from build123d import *

# Parameters (mm, degrees)
F0_R     = 6.35
F1_DEPTH = 12.7
F3_R     = 6.35
F4_DEPTH = 12.7


with BuildPart() as f1:
    # F0 (on Top) → F1 (new body)
    with BuildSketch(Plane.XY):
        with BuildLine():
            ThreePointArc((-163.4358839095, -121.5245512031), (-148.5569083937, -157.4455756873), (-112.6358839095, -172.3245512031))
            Line((-112.6358839095, -172.3245512031), (119.0192133605, -172.3245512031))
            ThreePointArc((119.0192133605, -172.3245512031), (154.9402378448, -157.4455756873), (169.8192133605, -121.5245512031))
            Line((169.8192133605, -121.5245512031), (169.8192133605, 115.6596517303))
            ThreePointArc((169.8192133605, 115.6596517303), (154.9402378448, 151.5806762145), (119.0192133605, 166.4596517303))
            Line((119.0192133605, 166.4596517303), (-112.6358839095, 166.4596517303))
            ThreePointArc((-112.6358839095, 166.4596517303), (-148.5569083937, 151.5806762145), (-163.4358839095, 115.6596517303))
            Line((-163.4358839095, 115.6596517303), (-163.4358839095, -121.5245512031))
        make_face()
        Polygon((-17.7260840714, -157.4455756873), (1.3239159286, -106.6455756873), (20.3739159286, -157.4455756873), align=None, mode=Mode.SUBTRACT)
        Polygon((-148.5569083937, -21.0277362994), (-148.5569083937, 17.0722637006), (-97.7569083937, 0.7111747481), align=None, mode=Mode.SUBTRACT)
        with Locations((1.3239159286, 0.7111747481)):
            Circle(F0_R, mode=Mode.SUBTRACT)
        Polygon((20.3739159286, 151.5806762145), (1.3239159286, 100.7806762145), (-17.7260840714, 151.5806762145), align=None, mode=Mode.SUBTRACT)
        Polygon((154.9402378448, -21.0277362994), (104.1402378448, 0.7111747481), (154.9402378448, 17.0722637006), align=None, mode=Mode.SUBTRACT)
    extrude(amount=F1_DEPTH)


with BuildPart() as f4:
    # F3 (on Top) → F4 (new body)
    with BuildSketch(Plane.XY):
        with BuildLine():
            ThreePointArc((-163.4358839095, -121.5245512031), (-148.5569083937, -157.4455756873), (-112.6358839095, -172.3245512031))
            Line((-112.6358839095, -172.3245512031), (119.0192133605, -172.3245512031))
            ThreePointArc((119.0192133605, -172.3245512031), (154.9402378448, -157.4455756873), (169.8192133605, -121.5245512031))
            Line((169.8192133605, -121.5245512031), (169.8192133605, 115.6596517303))
            ThreePointArc((169.8192133605, 115.6596517303), (154.9402378448, 151.5806762145), (119.0192133605, 166.4596517303))
            Line((119.0192133605, 166.4596517303), (-112.6358839095, 166.4596517303))
            ThreePointArc((-112.6358839095, 166.4596517303), (-148.5569083937, 151.5806762145), (-163.4358839095, 115.6596517303))
            Line((-163.4358839095, 115.6596517303), (-163.4358839095, -121.5245512031))
        make_face()
        with BuildLine():
            ThreePointArc((-68.5260840714, -21.0277362994), (-32.6050595871, -35.9067118152), (-17.7260840714, -71.8277362994))
            Line((-17.7260840714, -71.8277362994), (-17.7260840714, -106.6455756873))
            ThreePointArc((-17.7260840714, -106.6455756873), (-32.6050595871, -142.5666001716), (-68.5260840714, -157.4455756873))
            Line((-68.5260840714, -157.4455756873), (-97.7569083937, -157.4455756873))
            ThreePointArc((-97.7569083937, -157.4455756873), (-133.677932878, -142.5666001716), (-148.5569083937, -106.6455756873))
            Line((-148.5569083937, -106.6455756873), (-148.5569083937, -71.8277362994))
            ThreePointArc((-148.5569083937, -71.8277362994), (-133.677932878, -35.9067118152), (-97.7569083937, -21.0277362994))
            Line((-97.7569083937, -21.0277362994), (-68.5260840714, -21.0277362994))
        make_face(mode=Mode.SUBTRACT)
        Polygon((-17.7260840714, -157.4455756873), (1.3239159286, -106.6455756873), (20.3739159286, -157.4455756873), align=None, mode=Mode.SUBTRACT)
        with BuildLine():
            Line((71.1739159286, -21.0277362994), (104.1402378448, -21.0277362994))
            ThreePointArc((104.1402378448, -21.0277362994), (140.0612623291, -35.9067118152), (154.9402378448, -71.8277362994))
            Line((154.9402378448, -71.8277362994), (154.9402378448, -106.6455756873))
            ThreePointArc((154.9402378448, -106.6455756873), (140.0612623291, -142.5666001716), (104.1402378448, -157.4455756873))
            Line((104.1402378448, -157.4455756873), (71.1739159286, -157.4455756873))
            ThreePointArc((71.1739159286, -157.4455756873), (35.2528914443, -142.5666001716), (20.3739159286, -106.6455756873))
            Line((20.3739159286, -106.6455756873), (20.3739159286, -71.8277362994))
            ThreePointArc((20.3739159286, -71.8277362994), (35.2528914443, -35.9067118152), (71.1739159286, -21.0277362994))
        make_face(mode=Mode.SUBTRACT)
        Polygon((-148.5569083937, -21.0277362994), (-148.5569083937, 17.0722637006), (-97.7569083937, 0.7111747481), align=None, mode=Mode.SUBTRACT)
        with Locations((1.3239159286, 0.7111747481)):
            Circle(F3_R, mode=Mode.SUBTRACT)
        with BuildLine():
            ThreePointArc((-68.5260840714, 151.5806762145), (-32.6050595871, 136.7017006988), (-17.7260840714, 100.7806762145))
            Line((-17.7260840714, 100.7806762145), (-17.7260840714, 67.8722637006))
            ThreePointArc((-17.7260840714, 67.8722637006), (-32.6050595871, 31.9512392163), (-68.5260840714, 17.0722637006))
            Line((-68.5260840714, 17.0722637006), (-97.7569083937, 17.0722637006))
            ThreePointArc((-97.7569083937, 17.0722637006), (-133.677932878, 31.9512392163), (-148.5569083937, 67.8722637006))
            Line((-148.5569083937, 67.8722637006), (-148.5569083937, 100.7806762145))
            ThreePointArc((-148.5569083937, 100.7806762145), (-133.677932878, 136.7017006988), (-97.7569083937, 151.5806762145))
            Line((-97.7569083937, 151.5806762145), (-68.5260840714, 151.5806762145))
        make_face(mode=Mode.SUBTRACT)
        Polygon((20.3739159286, 151.5806762145), (1.3239159286, 100.7806762145), (-17.7260840714, 151.5806762145), align=None, mode=Mode.SUBTRACT)
        Polygon((154.9402378448, -21.0277362994), (104.1402378448, 0.7111747481), (154.9402378448, 17.0722637006), align=None, mode=Mode.SUBTRACT)
        with BuildLine():
            ThreePointArc((154.9402378448, 67.8722637006), (140.0612623291, 31.9512392163), (104.1402378448, 17.0722637006))
            Line((104.1402378448, 17.0722637006), (71.1739159286, 17.0722637006))
            ThreePointArc((71.1739159286, 17.0722637006), (35.2528914443, 31.9512392163), (20.3739159286, 67.8722637006))
            Line((20.3739159286, 67.8722637006), (20.3739159286, 100.7806762145))
            ThreePointArc((20.3739159286, 100.7806762145), (35.2528914443, 136.7017006988), (71.1739159286, 151.5806762145))
            Line((71.1739159286, 151.5806762145), (104.1402378448, 151.5806762145))
            ThreePointArc((104.1402378448, 151.5806762145), (140.0612623291, 136.7017006988), (154.9402378448, 100.7806762145))
            Line((154.9402378448, 100.7806762145), (154.9402378448, 67.8722637006))
        make_face(mode=Mode.SUBTRACT)
    extrude(amount=F4_DEPTH)


solid = f4.part
Source: CAD feature listing. Evaluate the final solid. Frame: model axes, mm. Round coordinates to 2 decimals unless told otherwise and drop trailing zeros. Loops run counter-clockwise (first coordinate to the right, second up) from the corner with the lowest first, then second, coordinate; pieces in that order, holes last. Notation, with made-up numbers: M 89,67 L 105,67 A21 ccw 105,103 Z; hole C 30.25,84.25 d11. An arc over 180 degrees is marked long. Return JSON: item names as keys, results as strings. Group by question number.
1. Section query D-D on x = -128.5. Output: boundary loops of the cut face in (y, z), and give its area (3 significant figures).
2. Section query A-A on x = -85.5. Output: boundary loops of the cut face in (y, z).
3. Mould query, pull axis Y, two halves, no side actions, for faces 1 (the face through (20.374, 84, 6)), 2 (the face through (155.333, 151.184, 6.261)). Classes: released by +Y, released by -Y, zero draft, split by the parting line, or undercut.
4. Section query B-B on y = -25. Output: boundary loops of the cut face in (x, z), and give its area (3 significant figures).
5. Section query C-C on y = 126. Output: boundary loops of the cut face in (x, z).
6. Material intervals for line 1 along Y through (x, z) = (-87, 2); line 2 along X through (y, z) = (-85.5, 5.25); line 3 along X through (y, z) = (-29, 10.5), sorted ascending. Write a range as from..to.
Checks:
{
 "1": {"outline": "M -169.78,0 L -147.09,0 L -147.09,12.7 L -169.78,12.7 Z; M -31.39,0 L -12.44,0 L -12.44,12.7 L -31.39,12.7 Z; M 10.61,0 L 27.43,0 L 27.43,12.7 L 10.61,12.7 Z; M 141.22,0 L 163.92,0 L 163.92,12.7 L 141.22,12.7 Z", "area": "1,030 mm²"},
 "2": {"outline": "M -172.32,0 L -157.45,0 L -157.45,12.7 L -172.32,12.7 Z; M -21.03,0 L 17.07,0 L 17.07,12.7 L -21.03,12.7 Z; M 151.58,0 L 166.46,0 L 166.46,12.7 L 151.58,12.7 Z"},
 "3": {"face 1": "undercut", "face 2": "released by +Y"},
 "4": {"outline": "M -163.44,0 L -117.45,0 L -117.45,12.7 L -163.44,12.7 Z; M -48.83,0 L 51.48,0 L 51.48,12.7 L -48.83,12.7 Z; M 123.83,0 L 169.82,0 L 169.82,12.7 L 123.83,12.7 Z", "area": "2,440 mm²"},
 "5": {"outline": "M -162.37,0 L -141.85,0 L -141.85,12.7 L -162.37,12.7 Z; M -24.43,0 L -8.13,0 L -8.13,12.7 L -24.43,12.7 Z; M 10.78,0 L 27.08,0 L 27.08,12.7 L 10.78,12.7 Z; M 148.24,0 L 168.76,0 L 168.76,12.7 L 148.24,12.7 Z"},
 "6": {"line 1": "y = -172.32..-157.45, -21.03..17.07, 151.58..166.46", "line 2": "x = -163.44..-148.56, -17.73..20.37, 154.94..169.82", "line 3": "x = -163.44..-125.08, -41.21..43.85, 131.46..169.82"}
}
